from build123d import *

# Parameters (mm, degrees)
BOSS_EXTRUDE1_DEPTH = 8
CUT_EXTRUDE2_DEPTH  = 8
BOSS_EXTRUDE2_START = 8
BOSS_EXTRUDE2_DEPTH = 8
BOSS_EXTRUDE3_DEPTH = 16
SKETCH8_R           = 2.165
CUT_EXTRUDE3_DEPTH  = 46.694096166


with BuildPart() as part:
    # Sketch1 → Boss-Extrude1 (new body)
    with BuildSketch(Plane.XY):
        with BuildLine():
            Line((-19.5, 13.830605225), (-19.5, 0))
            Line((-19.5, 0), (-28.9068116, 0))
            ThreePointArc((-28.9068116, 0), (0, 28.9068116), (28.9068116, 0))
            Line((28.9068116, 0), (23.9068116, 0))
            ThreePointArc((23.9068116, 0), (7.257851427, 22.778481809), (-19.5, 13.830605225))
        make_face()
    extrude(amount=BOSS_EXTRUDE1_DEPTH)

    # Sketch5 → Cut-Extrude2 (cut)
    with BuildSketch(Plane(origin=(0, 0, 0), x_dir=(-1, 0, 0), z_dir=(0, 0, -1))):
        Polygon((0, 0), (-18.650935532, 14.955876592), (-43.503762329, 22.442447281), (-58.13318285, -8.31229871), align=None)
    extrude(amount=-CUT_EXTRUDE2_DEPTH, mode=Mode.SUBTRACT)

    # Sketch6 → Boss-Extrude2 (add)
    with BuildSketch(Plane(origin=(0, 0, 0), x_dir=(-1, 0, 0), z_dir=(0, 0, -1)).offset(BOSS_EXTRUDE2_START)):
        with BuildLine():
            Line((-28.9068116, 0), (-18.11056, 0))
            ThreePointArc((-18.11056, 0), (0, 18.11056), (18.11056, 0))
            Line((18.11056, 0), (28.9068116, 0))
            ThreePointArc((28.9068116, 0), (0, 28.9068116), (-28.9068116, 0))
        make_face()
    extrude(amount=-BOSS_EXTRUDE2_DEPTH)

    # Sketch7 → Boss-Extrude3 (add, through all)
    with BuildSketch(Plane(origin=(0, 0, -8), x_dir=(-1, 0, 0), z_dir=(0, 0, -1))):
        with BuildLine():
            Line((28.9068116, 0), (38.11056, 0))
            Line((38.11056, 0), (38.11056, 5))
            Line((38.11056, 5), (28.471103893, 5))
            ThreePointArc((28.471103893, 5), (28.797678666, 2.509474109), (28.9068116, 0))
        make_face()
    extrude(amount=-BOSS_EXTRUDE3_DEPTH)

    # Sketch8 → Cut-Extrude3 (cut, through all)
    with BuildSketch(Plane(origin=(0, 5, 0), x_dir=(1, 0, 0), z_dir=(0, 1, 0))):
        with Locations(Location((-33.290831946, 0, 0), (0, 0, 270))):
            Circle(SKETCH8_R)
    extrude(amount=-CUT_EXTRUDE3_DEPTH, mode=Mode.SUBTRACT)


solid = part.part
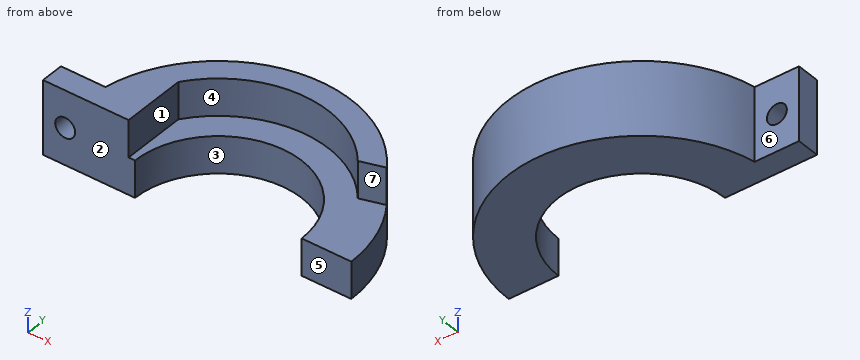
Check sheet for the modelled part. Datum: model origin and axes. Units: mm. Face numbers are marked on the shaded views. A direction names the side the tool comes from. Give positions to 0.01 mm unless a question says otherwise; leave off trailing zeros. Loops run counter-clockwise (first coordinate to the right, second up) from the corner with the lowest first, then second, coordinate; pieces in that order, holes last. Notation, with made-up numbers: M 10,19.5 L 50,19.5 A26 ccw 50,49.5 Z; hole C 58,-9.75 d11. An arc over 180 degrees is marked long. Return JSON: item names as keys, results as strings. Group by question number.
1. Thickness scan on L1, parallel to Y at x = -0.5, z = 4.25; L2, parallel to X at y = 7.5, z = -4; L3, parallel to X at y = 15.25, z = -7. Record the ranges inside material, lowest first.
2. Cross-section at C-C on y = 15.75. Record the boundary of the cut face in (x, z), plus the area to 3 significant figures.
3. Tool access check on the marked faces 4, 5, 6 and 7. Record the directions out of +Z, -Z, +X, -X, +Y, -Y that give a thin tool (end or side, any length) a straight path to the whole face; none if there is none.
4. Cross-section at B-B on z = 4.25. Record the boundary of the cut face in (x, y), plus the area to 3 significant figures.
5. Go/stop test with flat-tipped pins: pin 1 (2 mm diameter, centred on x = 10, z = 6, fed in from -Y); pin 2 (7.5 mm diameter, centred on x = -33.5, z = 0.5, fed in from +Y); pin 3 (5 mm diameter, centred on y = 3.5, z = -5.5, fed in from +X). Record where each tip stops, or that it passes through.
6. Cross-section at A-A on y = 3.25. Record the boundary of the cut face in (x, z) (3 decimals).
7. Mould release check, pull along X, two halves, no side actions. Record for the marked faces 1, 2 and 3: released by +X, released by -X, zero draft, split by the parting line, or undercut.
8. Cross-section at D-D on x = 0. Record the boundary of the cut face in (y, z).
Return value:
{
 "1": {"L1": "23.9 to 28.9", "L2": "-27.92 to -16.48, 16.48 to 27.92", "L3": "-24.56 to -9.77, 9.77 to 24.56"},
 "2": {"outline": "M -24.24,-8 L -8.94,-8 L -8.94,0 L -17.99,0 L -17.99,8 L -24.24,8 Z; M 8.94,-8 L 24.24,-8 L 24.24,0 L 21.29,0 L 21.29,8 L 17.99,8 L 17.99,0 L 8.94,0 Z", "area": "321 mm^2"},
 "3": {"face 4": "+Z, -Y", "face 5": "+Z, -Z, +X, -X, -Y", "face 6": "+Z, -Z, -X, +Y", "face 7": "+Z, +X, -Y"},
 "4": {"outline": "M -38.11,0 L -19.5,0 L -19.5,13.83 A23.91 cw 18.65,14.96 L 23.74,16.49 A28.91 ccw -28.47,5 L -38.11,5 Z", "area": "419 mm^2"},
 "5": {"pin 1": "y = 21.23", "pin 2": "y = 5", "pin 3": "x = 28.89"},
 "6": {"outline": "M -38.111,-8 L -17.817,-8 L -17.817,0 L -19.5,0 L -19.5,8 L -38.111,8 Z; M 17.817,-8 L 28.724,-8 L 28.724,0 L 17.817,0 Z; hole C -33.291,0 d4.33"},
 "7": {"face 1": "released by +X", "face 2": "zero draft", "face 3": "undercut"},
 "8": {"outline": "M 18.11,-8 L 28.91,-8 L 28.91,8 L 23.91,8 L 23.91,0 L 18.11,0 Z"}
}
